Autodesk Inventor part; units mm, degrees
ref_plane "YZ Plane" through (0, 0, 0) normal (1, 0, 0) x (0, 1, 0)
ref_plane "XZ Plane" through (0, 0, 0) normal (0, 1, 0) x (-1, 0, 0)
ref_plane "XY Plane" through (0, 0, 0) normal (0, 0, 1) x (1, 0, 0)
sketch "スケッチ1" plane through (0, 0, 0) normal (0, 1, 0) x (-1, 0, 0)
  line L0 (250, 100) -> (-250, 100)
  line L1 (-250, 100) -> (-250, -100)
  line L2 (-250, -100) -> (250, -100)
  line L3 (250, -100) -> (250, 100)
  point P0 (0, 0)
  dimension "d2" = 250
  dimension "d3" = 500
  dimension "d4" = 100
  dimension "d5" = 200
extrude "押し出し1" add sketch "スケッチ1" along normal blind 35
sketch "スケッチ2" plane through (-250, 0, 100) normal (0, 0, 1) x (1, 0, 0)
  line L0 (0, 35) -> (500, 35)
  line L1 (0, 0) -> (500, 0)
  arc A0 (0, 35) -> (90, 0) centre (90, 133.2143) ccw
  line L2 (0, 0) -> (0, 35)
  point P0 (250, 0)
  dimension "d8" = 90
extrude "押し出し2" cut sketch "スケッチ2" against normal through all
sketch "スケッチ5" plane through (-160, 0, 100) normal (0, 0, 1) x (1, 0, 0)
  arc A0 (-90, 35) -> (0, 0) centre (0, 133.2143) ccw
  line L0 (0, 0) -> (410, 0)
  arc A1 (-80.8544, 35) -> (0, 6) centre (0, 133.2143) ccw
  line L1 (0, 6) -> (54.4195, 6)
  line L2 (54.4195, 6) -> (410, 6)
  line L3 (-90, 35) -> (410, 35)
  line L4 (410, 0) -> (410, 35)
  point P0 (160, 0)
  point P1 (40, 35)
  dimension "d20" = 6
extrude "押し出し5" cut sketch "スケッチ5" against normal through all contours L3 L4 L2 L1 A1
sketch "スケッチ8" plane through (-160, 6, 100) normal (0, 1, 0) x (1, 0, 0)
  line L0 (210, 150) -> (160, 150)
  line L1 (410, 200) -> (410, 0)
  line L2 (0, 200) -> (410, 200)
  arc A0 (160, 150) -> (-90, 80) centre (160, -331.4286) ccw
  line L3 (-90, 200) -> (-90, 0)
  line L4 (-80.8544, 200) -> (0, 200)
  line L5 (-80.8544, 200) -> (-90, 200)
  line L6 (210, 156) -> (160, 156)
  arc A1 (160, 156) -> (-90, 87.005) centre (160, -331.4286) ccw
  line L7 (210, 150) -> (210, 156)
  line L8 (410, 0) -> (410, 200)
  line L9 (-90, 87.005) -> (-90, 80)
  point P0 (160, 100)
  dimension "d35" = 50
  dimension "d36" = 120
  dimension "d38" = 6
  dimension "d47" = 250
  dimension "d48" = 50
extrude "押し出し7" add sketch "スケッチ8" along normal up to surface (29 mm away)
delete faces "面を削除1" heal yes whole lump no faces at (-246.2129, 22.2141, 17.7225) (-250, 25.3333, 15.33) (-244.511, 6, 14.4766) (-246.2115, 22.2135, 10.7547)
sketch "スケッチ10" plane through (-160, 6, 100) normal (0, 1, 0) x (1, 0, 0)
  line L0 (410, 150) -> (410, 0)
  line L1 (410, 0) -> (0, 0)
  line L2 (410, 0) -> (410, 200)
  line L3 (410, 120) -> (10, 0)
  line L4 (0, 0) -> (410, 0)
  point P0 (160, 100)
  point P1 (210, 150)
  dimension "d43" = 400
  dimension "d44" = 120
extrude "押し出し9" cut sketch "スケッチ10" against normal through all
sketch "スケッチ11" plane through (250, 6, -100) normal (0, 0, -1) x (-1, 0, 0)
  line L0 (0, -6) -> (410, -6)
  arc A0 (410, -6) -> (500, 29) centre (410, 127.2143) ccw
  line L1 (0, -6) -> (0, 29)
  line L2 (0, 29) -> (500, 29)
  point P0 (250, -6)
extrude "押し出し10" add sketch "スケッチ11" against normal blind 6
sketch "スケッチ12" plane through (0, 0, 0) normal (0, 1, 0) x (-1, 0, 0)
  line L0 (250, -100) -> (250, 100)
  line L1 (250, 100) -> (0, 100)
  line L2 (0, 100) -> (0, 75)
  line L3 (0, 75) -> (250, 75)
  line L4 (250, 75) -> (250, 100)
  point P0 (0, 0)
  dimension "d51" = 25
extrude "押し出し11" cut sketch "スケッチ12" along normal through all
properties part number "endplate_ver2"
Input: part model. Units: mm. Frame: model coordinates. A direction names the side the tool comes from. Give positions to 0.01 mm unless a question says otherwise; leave off trailing zeros. Loops run counter-clockwise (first coordinate to the right, second up) from the corner with the lowest first, then second, coordinate; pieces in that order, holes last. Notation, with made-up numbers: (27.5, -37) -> (66.5, -37) arc R9 ccw to (66.5, -30) -> close; hole circle Ø2 at (80.5, 46.25). An arc over 180 degrees is marked (long way). Use a Markdown table: item, result.
Q1. First-contact query: P1, Ø5, axis at y = 14, z = 49, coming from the -X side; P2, Ø1.8, axis at y = 13.5, z = -51.5, coming from the +X side; P3, Ø3, axis at x = 89.5, z = 22.5, coming from the +Y side. Flat tips, straight axial feed; report the tip coordinate or a pass-through.
Entries:
| item | result |
|---|---|
| P1 | stops at x = -224.22 |
| P2 | stops at x = 50 |
| P3 | stops at y = 6 |
Q2. Section query C-C, the plane y = 12. Return the cut outline in (x, z), plus the area to 3 significant figures.
Entries:
| item | result |
|---|---|
| outline | (-215.26, -100) -> (250, -100) -> (250, -94) -> (-198.61, -94) -> (-198.61, -13.7) arc R487.43 ccw to (0, -56) -> (50, -56) -> (50, -50) -> (0, -50) arc R481.43 cw to (-198.61, -7.12) -> (-198.61, 75) -> (-215.26, 75) -> close |
| area | 7,130 mm² |
Q3. Access query for faces 4 (the flat face through (25, 20, -50)), 5 (the flat face through (25, 20, -56)), 6 (the cylindrical face through (-203.53, 13.68, -53.75)). Directions: +Z, -Z, +X, -X, +Y, -Y. A direction counts if a zero-diameter tool reaches every point of the face in a straight line with its end or side. Return the directions, or none.
Entries:
| item | result |
|---|---|
| face 4 | +Z, +X, +Y |
| face 5 | +X, +Y |
| face 6 | +Y |
Q4. Section query A-A, the plane x = 120.5. Return the cut outline in (y, z), plus the area to 3 significant figures.
Entries:
| item | result |
|---|---|
| outline | (0, -100) -> (35, -100) -> (35, -94) -> (6, -94) -> (6, 18.85) -> (0, 18.85) -> close |
| area | 887 mm² |
Q5. Section query B-B, the plane z = -75. Return the cut outline in (x, y), plus the area to 3 significant figures.
Entries:
| item | result |
|---|---|
| outline | (-250, 35) arc R133.21 ccw to (-160, 0) -> (250, 0) -> (250, 6) -> (-160, 6) arc R127.21 cw to (-240.85, 35) -> close |
| area | 3,020 mm² |
Q6. Ray query, probe 1 along Z at (x, y) = (9, 18.5); probe 2 along Y at (x, z) = (-17.5, 44.5); probe 3 along Z at (x, y) = (168.5, 21.5). Return the intervals inside material, ascending. Write a range as from..to.
Entries:
| item | result |
|---|---|
| probe 1 | z = -100..-94, -56..-50 |
| probe 2 | y = 0..6 |
| probe 3 | z = -100..-94 |
Q7. Pull-direction query (Z, two-part tool) for faces 1 (the flat face through (-158, 4, 75)), 2 (the flat face through (8, 21, -94)), 3 (the flat face through (-112, 35, -39)); classes: pulls with the +Z half, pulls with the -Z half, needs draft (parallel to the pull), parting line crosses it, or undercut.
Entries:
| item | result |
|---|---|
| face 1 | pulls with the +Z half |
| face 2 | undercut |
| face 3 | needs draft |
Q8. Section query D-D, the plane x = -83. Return the cut outline in (y, z).
Entries:
| item | result |
|---|---|
| outline | (0, -100) -> (35, -100) -> (35, -94) -> (6, -94) -> (6, -48.88) -> (35, -48.88) -> (35, -42.79) -> (6, -42.79) -> (6, 75) -> (0, 75) -> close |
